```python
from build123d import *

# Parameters (mm, degrees)
SKETCH1_R          = 14.975
EXTRUDE1_DEPTH     = 12
SKETCH2_R          = 15
EXTRUDE2_DEPTH     = 11
SKETCH3_R          = 17.5
EXTRUDE3_DEPTH     = 10
SKETCH4_R          = 10
EXTRUDE4_DEPTH     = 24
SKETCH5_R          = 9.5
EXTRUDE5_DEPTH     = 1.3
SKETCH6_R          = 10
EXTRUDE6_DEPTH     = 25
SKETCH7_R          = 9
EXTRUDE7_DEPTH     = 36.5
SKETCH8_R          = 7.660195653
EXTRUDE8_DEPTH     = 15.5
SKETCH9_W          = 5
SKETCH9_H          = 5.185185185
CUT_EXTRUDE1_DEPTH = 14.5
FILLET1_R          = 2.5
CHAMFER1_SIZE      = 1.5
SKETCH10_W         = 6
SKETCH10_H         = 18
CUT_EXTRUDE2_DEPTH = 3
FILLET2_R          = 3
CUT_EXTRUDE3_DEPTH = 3
FILLET3_R          = 3
CHAMFER2_SIZE      = 1.5


with BuildPart() as part:
    # Sketch1 → Extrude1 (new body)
    with BuildSketch(Plane.XY):
        Circle(SKETCH1_R)
    extrude(amount=-EXTRUDE1_DEPTH)

    # Sketch2 → Extrude2 (add)
    with BuildSketch(Plane(origin=(0, 0, -12), x_dir=(-1, 0, 0), z_dir=(0, 0, -1))):
        Circle(SKETCH2_R)
    extrude(amount=EXTRUDE2_DEPTH)

    # Sketch3 → Extrude3 (add)
    with BuildSketch(Plane(origin=(0, 0, -23), x_dir=(-1, 0, 0), z_dir=(0, 0, -1))):
        Circle(SKETCH3_R)
    extrude(amount=EXTRUDE3_DEPTH)

    # Sketch4 → Extrude4 (add)
    with BuildSketch(Plane(origin=(0, 0, -33), x_dir=(-1, 0, 0), z_dir=(0, 0, -1))):
        Circle(SKETCH4_R)
    extrude(amount=EXTRUDE4_DEPTH)

    # Sketch5 → Extrude5 (add)
    with BuildSketch(Plane(origin=(0, 0, -57), x_dir=(-1, 0, 0), z_dir=(0, 0, -1))):
        Circle(SKETCH5_R)
    extrude(amount=EXTRUDE5_DEPTH)

    # Sketch6 → Extrude6 (add)
    with BuildSketch(Plane(origin=(0, 0, -58.3), x_dir=(-1, 0, 0), z_dir=(0, 0, -1))):
        Circle(SKETCH6_R)
    extrude(amount=EXTRUDE6_DEPTH)

    # Sketch7 → Extrude7 (add)
    with BuildSketch(Plane(origin=(0, 0, -83.3), x_dir=(-1, 0, 0), z_dir=(0, 0, -1))):
        Circle(SKETCH7_R)
    extrude(amount=EXTRUDE7_DEPTH)

    # Sketch8 → Extrude8 (add)
    with BuildSketch(Plane(origin=(0, 0, -119.8), x_dir=(-1, 0, 0), z_dir=(0, 0, -1))):
        Circle(SKETCH8_R)
    extrude(amount=EXTRUDE8_DEPTH)

    # Sketch9 → Cut-Extrude1 (cut)
    with BuildSketch(Plane.XY):
        with Locations((0, 15.292592593)):
            Rectangle(SKETCH9_W, SKETCH9_H)
    extrude(amount=-CUT_EXTRUDE1_DEPTH, mode=Mode.SUBTRACT)

    # Fillet1
    fillet1_edges = [part.edges().sort_by_distance(p)[0] for p in [
        (2.5, 13.745099729, -14.5),
        (-2.5, 13.745099729, -14.5),
    ]]
    fillet(fillet1_edges, radius=FILLET1_R - 0.0001)  # a hair under: the kernel refuses the full size

    # Chamfer1
    chamfer1_edges = [part.edges().sort_by_distance(p)[0] for p in [
        (0, -14.975, 0),
    ]]
    chamfer(chamfer1_edges, length=CHAMFER1_SIZE)

    # Sketch10 → Cut-Extrude2 (cut)
    with BuildSketch(Plane(origin=(0, 10, 0), x_dir=(-1, 0, 0), z_dir=(0, 1, 0))):
        with Locations((0, -44)):
            Rectangle(SKETCH10_W, SKETCH10_H)
    extrude(amount=-CUT_EXTRUDE2_DEPTH, mode=Mode.SUBTRACT)

    # Fillet2
    fillet2_edges = [part.edges().sort_by_distance(p)[0] for p in [
        (3, 8.269696007, -53),
        (-3, 8.269696007, -53),
        (-3, 8.269696007, -35),
        (3, 8.269696007, -35),
    ]]
    fillet(fillet2_edges, radius=FILLET2_R - 0.0001)  # a hair under: the kernel refuses the full size

    # Sketch11 → Cut-Extrude3 (cut)
    with BuildSketch(Plane(origin=(0, 9, 0), x_dir=(-1, 0, 0), z_dir=(0, 1, 0))):
        Polygon((-3.005512872, -84.3), (2.996762617, -84.3), (2.994487128, -106.299999882), (-3.005512872, -106.3), align=None)
    extrude(amount=-CUT_EXTRUDE3_DEPTH, mode=Mode.SUBTRACT)

    # Fillet3
    fillet3_edges = [part.edges().sort_by_distance(p)[0] for p in [
        (-2.994487128, 7.243614227, -106.299999882),
        (3.005512872, 7.241665132, -106.3),
        (3.005512872, 7.241665132, -84.3),
        (-2.996762617, 7.243212634, -84.3),
    ]]
    fillet(fillet3_edges, radius=FILLET3_R)

    # Chamfer2
    chamfer2_edges = [part.edges().sort_by_distance(p)[0] for p in [
        (7.660195653, 0, -135.3),
    ]]
    chamfer(chamfer2_edges, length=CHAMFER2_SIZE)


solid = part.part
```
Geometry: final body of the model. Coordinates: model frame, mm. A direction names the side the tool comes from. Round coordinates to 2 decimals unless told otherwise and drop trailing zeros. Order: outer loops, then holes, each group sorted by start corner. A loop starts at its lowest first (then second) coordinate and runs counter-clockwise, first axis right, second up. Notation, with made-up numbers: M -35.75,40 L 22.25,40 A16 ccw 22.25,61 Z; hole C -22,25.25 d4. An arc over 180 degrees is marked long. Use one line per item in the form item = value. Start each with the question number.
Q1. Cut plane A-A (z = -60). Return loops of the section in (x, y).
Q2. Cut plane B-B (z = -91). Return loops of the section in (x, y).
Q3. Material intervals for line 1 (Z direction, x = 9.5, y = -13); line 2 (Z direction, x = 2.5, y = 10); line 3 (X direction, y = -0.5, z = -40.5), sorted ascending. Write a range as [from, to].
Q4. Pin query (flat end, axial travel): pin 1 Ø5 at (x, z) = (1, -92.5) entering from +Y; pin 2 Ø1 at (x, z) = (-1.5, -96) entering from -Y; pin 3 Ø5 at (x, z) = (-1, -47.5) entering from +Y; pin 4 Ø1 at (x, z) = (-11, -79.5) entering from -Y. Return the tip coordinate at first contact, or that it passes through.
Q5. Access query for faces 1 (the face through (3, 8, -44)), 2 (the face through (13.887, -10.648, -27.93)), 3 (the face through (1.951, -8.786, -101.294)), 4 (the face through (-0.623, -14.962, -6.676)), 5 (the face through (-1.748, 13.866, -13.787)). Directions: +Z, -Z, +X, -X, +Y, -Y. A direction counts if a zero-diameter tool reaches every point of the face in a straight line with its end or side. Return the directions, or none.
Q6. Mould query, pull axis X, two halves, no side actions, for faces 6 (the face through (2.17, -9.76, -44.83)), 7 (the face through (-3, 8, -44)), 8 (the face through (2.1, 8.48, -52.14)), 9 (the face through (-7, 4, -119.8)). Classes: +X half, -X half, draft (parallel to the pull), parting line (faces both ways), or undercut.
Geometry results:
q1.outline = C 0,0 d20
q2.outline = M -3,6 L -3,8.49 A9 ccw long 3.01,8.48 L 3.01,6 Z
q3.line_1 = [-33, -23]
q3.line_2 = [-33, 0]
q3.line_3 = [-9.99, 9.99]
q4.pin_1 = 8.48
q4.pin_2 = -8.94
q4.pin_3 = 9.54
q4.pin_4 = through
q5.face_1 = +Y
q5.face_2 = +Z, -Z
q5.face_3 = -Z
q5.face_4 = +Z
q5.face_5 = +Z, +Y
q6.face_6 = parting line
q6.face_7 = undercut
q6.face_8 = undercut
q6.face_9 = draft
